Input: dimensioned drawing with shaded views. Units: mm. Origin: part minimum x, y, z. A direction names the side the tool comes from. Coordinates: 2 decimals unless noted, no trailing zeros. Loops run counter-clockwise (first coordinate to the right, second up) from the corner with the lowest first, then second, coordinate; pieces in that order, holes last.
(1) Mould query, pull axis Z, two halves, no side actions, for the marked faces 4, 5 and 6. Classes: released by +Z, released by -Z, zero draft, split by the parting line, or undercut.
(2) Section B-B, the plane z = 6. Return loops of the section in (x, y), then the cut area to 3 significant figures.
(3) Section A-A, the plane y = 3.5. Return loops of the section in (x, z).
(4) Section C-C, the plane x = 4.25. Return loops of the section in (y, z), then the cut area to 3 significant figures.
(5) Line query: L1, parallel to Y at x = 4.55, z = 9; L2, parallel to X at y = 17.5, z = 6.5; L3, parallel to Z at x = 0.5, y = 15.25. Output: solid intervals per line, ascending.
(6) Section D-D, the plane z = 8.75. Return loops of the section in (x, y).
(7) Set-up query: the marked faces 1, 2 and 3. Return all of +Z, -Z, +X, -X, +Y, -Y with unobstructed straight access to the full face (end or side cutting, diameter ignored); none if empty.
(8) Contact query for flat-ended pins moving along their axis: P1, Ø1.5, axis at y = 10, z = 4.5, coming from the +X side; P2, Ø2.5, axis at y = 3.5, z = 9, coming from the +X side; P3, Ø4, axis at x = 1, y = 9, coming from the +Z side; P4, Ø6, axis at y = 9, z = 7, coming from the -X side. Output: stop coordinate, or through.
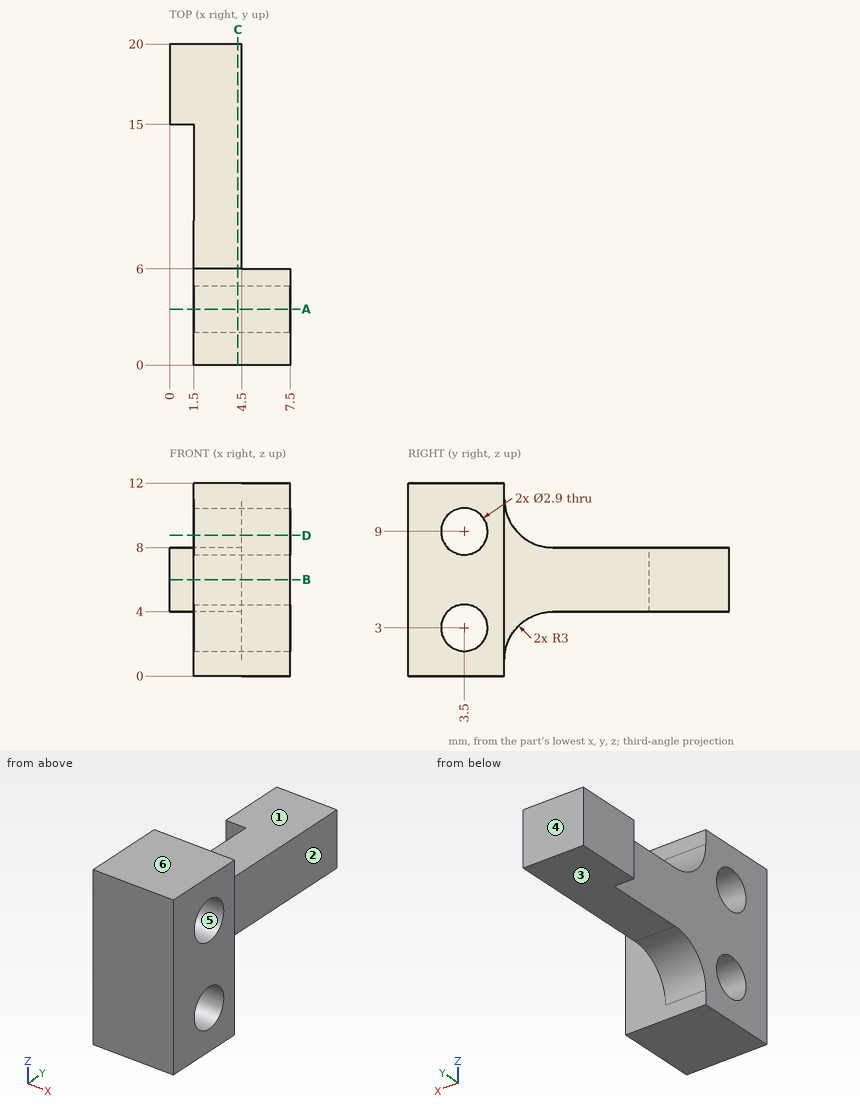
Report:
1. face 4: zero draft
1. face 5: undercut
1. face 6: released by +Z
2. outline: (0, 15) - (1.5, 15) - (1.5, 0) - (7.5, 0) - (7.5, 6) - (4.5, 6) - (4.5, 20) - (0, 20) - close
2. area: 85.5 mm2
3. outline: (1.5, 0) - (7.5, 0) - (7.5, 1.55) - (1.5, 1.55) - close; (1.5, 4.45) - (7.5, 4.45) - (7.5, 7.55) - (1.5, 7.55) - close; (1.5, 10.45) - (7.5, 10.45) - (7.5, 12) - (1.5, 12) - close
4. outline: (0, 0) - (6, 0) - (6, 1) arc R3 cw to (9, 4) - (20, 4) - (20, 8) - (9, 8) arc R3 cw to (6, 11) - (6, 12) - (0, 12) - close; hole circle Ø2.9 at (3.5, 3); hole circle Ø2.9 at (3.5, 9)
4. area: 119 mm2
5. L1: y = 0 to 2.05, 4.95 to 6
5. L2: x = 0 to 4.5
5. L3: z = 4 to 8
6. outline: (1.5, 0) - (7.5, 0) - (7.5, 2.07) - (1.5, 2.07) - close; (1.5, 4.93) - (7.5, 4.93) - (7.5, 6) - (4.5, 6) - (4.5, 7.02) - (1.5, 7.02) - close
7. face 1: +Z, +X, -X, +Y
7. face 2: +Z, -Z, +X, +Y
7. face 3: -Z, +X, -X, +Y
8. P1: stops at x = 4.5
8. P2: passes through
8. P3: stops at z = 8.71
8. P4: stops at x = 1.5
